The listing builds one solid part. Answer for the finished solid, in the listing's coordinates (mm). Face numbers are marked on the shaded views. Give positions to 0.01 mm unless a question says otherwise; leave off trailing zeros. Order: outer loops, then holes, each group sorted by start corner. A loop starts at its lowest first (then second) coordinate and runs counter-clockwise, first axis right, second up. Notation, with made-up numbers: (-29.5, -2) - (-12.5, -2) arc R21 ccw to (-12.5, 28) - close; hole circle Ø10 at (-9, 30.5). An arc over 180 degrees is marked (long way). Answer in a Markdown table with one row per item.
Autodesk Inventor part; units mm, degrees
ref_plane "YZ Plane" through (0, 0, 0) normal (1, 0, 0) x (0, 1, 0)
ref_plane "XZ Plane" through (0, 0, 0) normal (0, 1, 0) x (-1, 0, 0)
ref_plane "XY Plane" through (0, 0, 0) normal (0, 0, 1) x (1, 0, 0)
sketch "Sketch1" plane through (0, 0, 0) normal (0, 0, 1) x (1, 0, 0)
  arc A0 (53.8057, 7.6214) -> (60.8401, 7.187) centre (57.3363, 7.6214) ccw
  arc A1 (55.1426, 20.9078) -> (50.5197, 15.5843) centre (52.9772, 18.1193) ccw
  arc A2 (53.8057, 7.6214) -> (50.5197, 15.5843) centre (42.9913, 7.8181) ccw
  arc A3 (60.8401, 7.187) -> (55.1426, 20.9078) centre (45.9242, 9.0366) ccw
  dimension "d3" = 7.0612
  dimension "d4" = 7.0612
extrude "Extrusion1" add sketch "Sketch1" along normal blind 5.08
fillet "Fillet1" radius 0.635 4 edges at (57.1187, 4.0975, 5.08) (50.3114, 20.4341, 5.08) (52.9896, 11.9441, 5.08) (59.8052, 14.8006, 5.08)
sketch "Sketch2" plane through (0, 0, 5.08) normal (0, 0, 1) x (1, 0, 0)
  line L0 (55.3489, 14.773) -> (60.8716, 14.773) construction
  line L1 (60.8716, 14.773) -> (60.8716, 8.0828) construction
  line L2 (60.8716, 8.0828) -> (55.3489, 8.0828) construction
  line L3 (55.3489, 8.0828) -> (55.3489, 14.773) construction
  line L4 (56.5567, 11.725) -> (56.3245, 11.725)
  line L5 (56.3245, 11.725) -> (55.954, 12.9378)
  line L6 (55.954, 12.9378) -> (55.5761, 11.725)
  line L7 (55.5761, 11.725) -> (55.3563, 11.725)
  line L8 (55.3563, 11.725) -> (55.8429, 13.2514)
  line L9 (55.8429, 13.2514) -> (55.3711, 14.773)
  line L10 (55.3711, 14.773) -> (55.6033, 14.773)
  line L11 (55.6033, 14.773) -> (55.9664, 13.58)
  line L12 (55.9664, 13.58) -> (56.3369, 14.773)
  line L13 (56.3369, 14.773) -> (56.5567, 14.773)
  line L14 (56.5567, 14.773) -> (56.0775, 13.2712)
  line L15 (56.0775, 13.2712) -> (56.5567, 11.725)
  point P0 (0, 0)
extrude "Extrusion2" cut sketch "Sketch2" against normal blind 0.0635
properties part number "X Button"
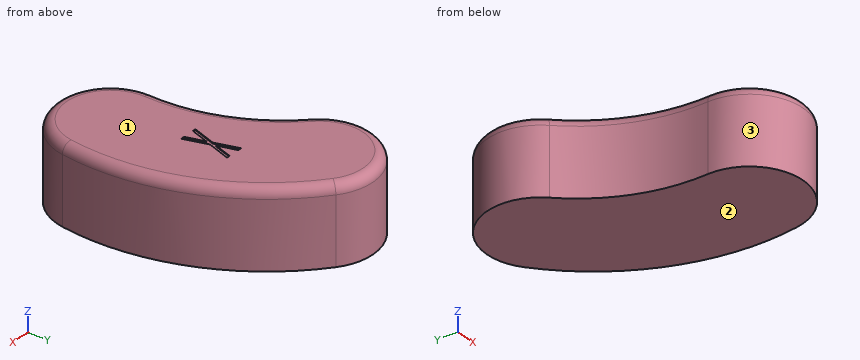
Item 1: Consider line 1 (Y direction, x = 55.75, z = 2.55); line 2 (Y direction, x = 56.75, z = 1.3); line 3 (X direction, y = 20, z = 0.35). Determine where each line is inside the solid, lowest interval first.
Answer block:
| item | result |
|---|---|
| line 1 | 4.47 to 20.41 |
| line 2 | 4.14 to 19.46 |
| line 3 | 49.99 to 56.21 |
Item 2: This flat-tipped pin is pushed along its axis until it touches: P1, Ø1.5, axis at y = 17, z = 3, coming from the +X side. Where does it stop, or does it pass through?
Answer block:
| item | result |
|---|---|
| P1 | x = 59.11 |
Item 3: Find section A-A on z = 0.9. Write down the section's boundary in (x, y).
Answer block:
| item | result |
|---|---|
| outline | (50.52, 15.58) arc R10.82 cw to (53.81, 7.62) arc R3.53 ccw to (60.84, 7.19) arc R15.03 ccw to (55.14, 20.91) arc R3.53 ccw to start |
Item 4: Find section B-B on z = 4.7. Write down the section's boundary in (x, y), then the cut area to 3 significant figures.
Answer block:
| item | result |
|---|---|
| outline | (50.56, 15.62) arc R10.87 cw to (53.86, 7.62) arc R3.48 ccw to (60.79, 7.19) arc R14.98 ccw to (55.11, 20.87) arc R3.48 ccw to start |
| area | 123 mm² |
Item 5: Determine the mould class of the marked faces 1, 2 and 3 for opening direction Z: pulls with the +Z half, pulls with the -Z half, needs draft (parallel to the pull), parting line crosses it, or undercut.
Answer block:
| item | result |
|---|---|
| face 1 | pulls with the +Z half |
| face 2 | pulls with the -Z half |
| face 3 | needs draft |
